```python
from build123d import *


# Not quite as in the source:
# - ends of sketch curves that miss each other by under 0.0002 mm in the source are joined
# - the dataset's text gives a spline's control points without its knots; the knots are read off the source's solid


with BuildPart() as f1:
    # F0 (on Front) → F1 (revolve)
    with BuildSketch(Plane.XZ):
        with BuildLine():
            Line((50.8, -68.5799818198), (0, -68.5799818198))
            Line((0, -68.5799818198), (0, -74.9299818198))
            Line((0, -74.9299818198), (57.15, -74.9299818198))
            Line((57.15, -74.9299818198), (57.15, 1.6272e-06))
            add(Edge.make_bspline(
                [(57.15, 1.6272e-06), (57.1499999994, 0.7047113918), (57.0598999162, 2.103273417), (56.6515693983, 4.1275628276), (55.9891831776, 6.0294834035), (55.1137080803, 7.7693366077), (54.0770742303, 9.3282529906), (52.5451803539, 11.1692858227), (50.4535495865, 13.0673465504), (47.8521882716, 14.8916410503), (45.252819746, 16.425180894), (42.7316484966, 17.7782729868), (40.3709871587, 19.0241328449), (38.6175601714, 20.0091031011), (37.3964709607, 20.7693815862), (36.5848410934, 21.3222974779), (35.889165019, 21.8521978188), (35.3187701783, 22.3490647419), (34.9484904994, 22.7282804416), (34.7161027204, 23.0004508821), (34.5495368253, 23.2155139733), (34.3902675999, 23.4425507333), (34.1858485185, 23.7641041974), (33.8467702825, 24.3818175191), (33.4109284532, 25.4497498628), (32.9816573877, 27.0498729284), (32.6545525856, 28.932648506), (32.411932376, 31.0443557544), (32.2145322917, 33.3333465292), (32.0061617084, 35.7596304469), (31.7139430509, 38.2985913452), (31.3207822666, 40.5019809383), (30.8480072544, 42.315454933), (30.4671278129, 43.4684021236), (30.0993683091, 44.3969660699), (29.7863286696, 45.0992011119), (29.4431534601, 45.7843141536), (28.9514880524, 46.6664553198), (28.2759351057, 47.710924054), (27.0873755974, 49.2504932123), (25.4420689363, 50.9266202701), (23.3260377998, 52.5809069603), (21.1425673416, 53.9478206558), (18.9367386048, 55.0958122319), (16.73909063, 56.0833338186), (15.292731043, 56.6675944469), (14.5776358142, 56.9480177287), (14.5734167567, 56.9496719276)],
                knots=[1.95e-08, 1.95e-08, 1.95e-08, 1.95e-08, 0.015625, 0.03125, 0.046875, 0.0625, 0.078125, 0.09375, 0.125, 0.15625, 0.1875, 0.21875, 0.25, 0.28125, 0.296875, 0.3125, 0.328125, 0.34375, 0.359375, 0.3671875, 0.375, 0.3828125, 0.390625, 0.40625, 0.4375, 0.46875, 0.5, 0.53125, 0.5625, 0.59375, 0.625, 0.65625, 0.671875, 0.6875, 0.6953125, 0.703125, 0.7109375, 0.71875, 0.734375, 0.75, 0.78125, 0.8125, 0.84375, 0.875, 0.90625, 0.9375, 0.9376854849, 0.9376854849, 0.9376854849, 0.9376854849], degree=3))
            Line((14.5734167567, 56.9496719276), (14.5734162837, 71.0851369262))
            Line((14.5734162837, 71.0851369262), (3.6679329351, 71.0851369262))
            Line((3.6679329351, 71.0851369262), (3.6679329351, 64.7351369262))
            Line((3.6679329351, 64.7351369262), (8.2234162837, 64.7351369262))
            Line((8.2234162837, 64.7351369262), (8.2234162837, 52.5710880756))
            add(Edge.make_bspline(
                [(50.8, 0), (50.8000016062, 10.1355050023), (21.8530368998, 13.6006812311), (29.227455035, 45.4185092323), (14.6406068987, 50.1267635615), (8.2234162837, 52.5710880756)],
                knots=[0, 0, 0, 0, 0.3637012491, 0.7015500616, 1, 1, 1, 1], degree=3))
            Line((50.8, 0), (50.8, -68.5799818198))
        make_face()
    revolve(axis=Axis((0, 0, -71.7549818198), (0, 0, -1)))


solid = f1.part
```
CAD build for the part. Positions are in the model's coordinates, mm. A direction names the side the tool comes from. Round coordinates to 2 decimals unless told otherwise and drop trailing zeros. Order: outer loops, then holes, each group sorted by start corner. A loop starts at its lowest first (then second) coordinate and runs counter-clockwise, first axis right, second up. Notation, with made-up numbers: (18.25, -4.5) - (73.25, -4.5) arc R28 cw to (73.25, 33.5) - close; hole circle Ø8 at (-23.5, -1). An arc over 180 degrees is marked (long way). Answer as CSV lines item,"result". Start each with the question number.
1. Pull direction Z, two halves, no side cores. Call faces 4 (the face through (-4, 2, 64.735)), 5 (the face through (1, -1, -74.93)), 6 (the face through (-57.095, -2.513, -36.94)): +Z half, -Z half, draft (parallel to the pull), parting line (faces both ways), or undercut.
2. Drill centre lines: L1, parallel to Z at x = 1.5, y = 6; L2, parallel to Y at x = 0, z = 67.75; L3, parallel to Y at x = 0, z = -41.5. Where is each one in solid material? Low to high. Write a range as [from, to].
3. Tool access for faces 1 (the face through (-11.012, 49.592, -34.77)), 2 (the face through (3, 3, 71.085)), 3 (the face through (-3.159, 14.227, 64.116)): list every direction of +Z, -Z, +X, -X, +Y, -Y with a clear straight run to the whole face (end or side of a thin tool).
4. Saw through at A-A, the plane z = -64. Write the cut outline in (x, y), and give its area (3 significant figures).
5. Pin check, flat tips, straight feed: pin 1 (6 mm diameter, centred on x = 35, z = 16, fed in from -Y); pin 2 (1.5 mm diameter, centred on y = -16, z = 23, fed in from -X); pin 3 (6 mm diameter, centred on x = 0, y = 0, fed in from +Z). Stop position of each tip, or through.
Model answer:
1,face 4,"undercut"
1,face 5,"-Z half"
1,face 6,"draft"
2,L1,"z = [-74.93, -68.58], [64.74, 71.09]"
2,L2,"y = [-14.57, -3.67], [3.67, 14.57]"
2,L3,"y = [-57.15, -50.8], [50.8, 57.15]"
3,face 1,"none"
3,face 2,"+Z, +X, -X, +Y, -Y"
3,face 3,"+Z"
4,outline,"circle Ø114.3 at (0, 0); hole circle Ø101.6 at (0, 0)"
4,area,"2,150 mm²"
5,pin 1,"stops at y = -37.01"
5,pin 2,"stops at x = -31.7"
5,pin 3,"stops at z = -68.58"
